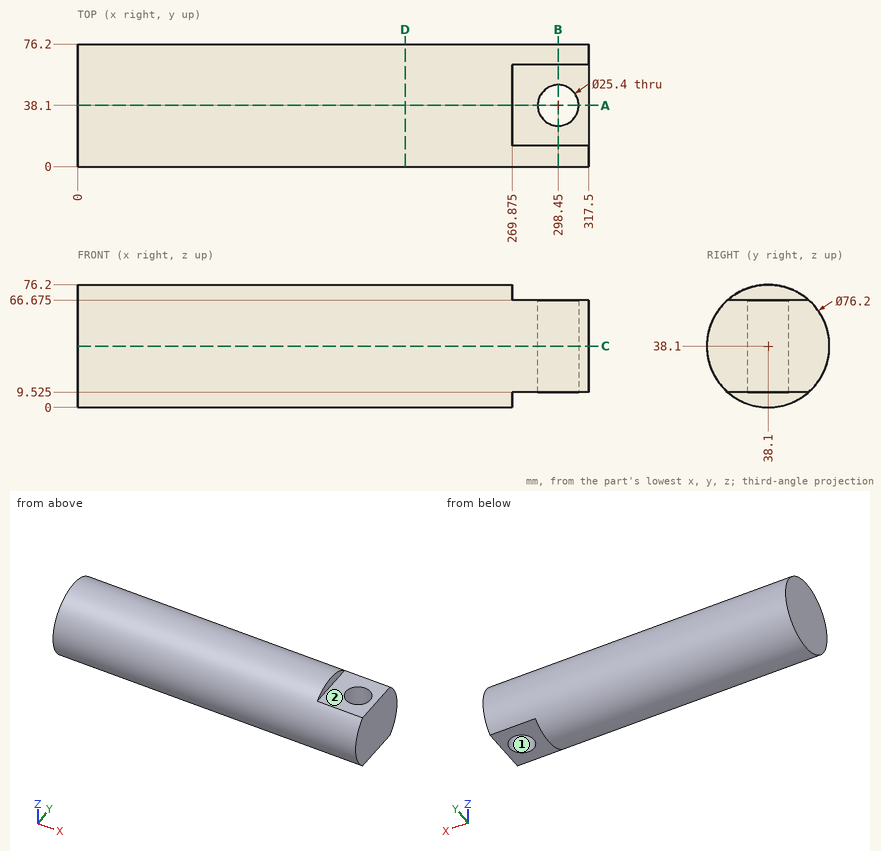
Check sheet for the drawn part. Datum: minimum x, y, z corner. Units: mm. A direction names the side the tool comes from. Give positions to 0.01 mm unless a question says otherwise; leave off trailing zeros. Order: outer loops, then holes, each group sorted by start corner. A loop starts at its lowest first (then second) coordinate and runs counter-clockwise, first axis right, second up. Notation, with made-up numbers: (45.25, 50) -> (77.25, 50) arc R13 ccw to (77.25, 54) -> close; hole circle Ø5 at (54, 1). An arc over 180 degrees is marked (long way). Return JSON: item names as keys, results as strings.
1. Go/stop test with flat-tipped pins: P1, Ø3, axis at x = 153, z = 54, coming from the -Y side; P2, Ø8, axis at x = 168.5, y = 68, coming from the -Z side; P3, Ø1, axis at x = 142.5, z = 22.5, coming from the -Y side; P4, Ø7.5, axis at y = 27, z = 7, coming from the +X side. Record where each tip stops, or that it passes through.
From the geometry:
{"P1": "y = 2.83", "P2": "z = 10.16", "P3": "y = 3.12", "P4": "x = 317.5"}
2. Set-up check for the marked faces 1 and 2: record each of +Z, -Z, +X, -X, +Y, -Y from which the full face is reachable in a straight line by a thin tool's end or side.
From the geometry:
{"face 1": "+Z, -Z", "face 2": "+Z, +X, +Y, -Y"}
3. Cross-section at D-D, the plane x = 203.5. Record the cut outline in (y, z), plus the area to 3 significant figures.
From the geometry:
{"outline": "circle Ø76.2 at (38.1, 38.1)", "area": "4,560 mm^2"}
4. Material ranges on probe 1 along X at (y, z) = (38, 39); probe 2 along X at (y, z) = (33, 51.5); probe 3 along X at (y, z) = (45, 6) (3 decimals), recorded low to high. Write a range as [from, to].
From the geometry:
{"probe 1": "[0, 285.75], [311.15, 317.5]", "probe 2": "[0, 286.82], [310.08, 317.5]", "probe 3": "[0, 269.875]"}
5. Cross-section at B-B, the plane x = 298.45. Record the cut outline in (y, z) (3 decimals), plus the area to 3 significant figures.
From the geometry:
{"outline": "(12.899, 9.525) -> (25.4, 9.525) -> (25.4, 66.675) -> (12.899, 66.675) arc R38.1 ccw to start; (50.8, 9.525) -> (63.301, 9.525) arc R38.1 ccw to (63.301, 66.675) -> (50.8, 66.675) -> close", "area": "2,450 mm^2"}
6. Cross-section at C-C, the plane z = 38.1. Record the cut outline in (x, y).
From the geometry:
{"outline": "(0, 0) -> (317.5, 0) -> (317.5, 76.2) -> (0, 76.2) -> close; hole circle Ø25.4 at (298.45, 38.1)"}
7. Cross-section at A-A, the plane y = 38.1. Record the cut outline in (x, z) (3 decimals).
From the geometry:
{"outline": "(0, 0) -> (269.875, 0) -> (269.875, 9.525) -> (285.75, 9.525) -> (285.75, 66.675) -> (269.875, 66.675) -> (269.875, 76.2) -> (0, 76.2) -> close; (311.15, 9.525) -> (317.5, 9.525) -> (317.5, 66.675) -> (311.15, 66.675) -> close"}
